```python
from build123d import *

# Parameters (mm, degrees)
BOSS_EXTRUDE1_DEPTH = 5
FILLET1_R           = 1


with BuildPart() as part:
    # Sketch1 → Boss-Extrude1 (new body)
    with BuildSketch(Plane.XY):
        Polygon((0, 0), (133, 0), (133, 12.3), (123.25, 12.3), (123.25, 10.3), (128.25, 10.3), (128.25, 5), (10, 5), (10, 10.3), (19, 10.3), (19, 30), (0, 30), align=None)
    extrude(amount=BOSS_EXTRUDE1_DEPTH)

    # Mirror1: part across plane


with BuildPart() as part_1:
    add(part.part)
    add(part.part.mirror(Plane(origin=(133, 12.3, 5), x_dir=(0, 0, 1), z_dir=(-1, 0, 0))))

    # Fillet1
    fillet1_edges = [part_1.edges().sort_by_distance(p)[0] for p in [
        (0, 30, 2.5),
        (19, 30, 2.5),
        (19, 10.3, 2.5),
        (0, 0, 2.5),
        (266, 0, 2.5),
        (247, 10.3, 2.5),
        (247, 30, 2.5),
        (266, 30, 2.5),
    ]]
    fillet(fillet1_edges, radius=FILLET1_R)


solid = part_1.part
```
Design review of the part built by this model. Coordinates are the model's own, in mm. A direction names the side the tool comes from. Give positions to 0.01 mm unless a question says otherwise; leave off trailing zeros. Loops run counter-clockwise (first coordinate to the right, second up) from the corner with the lowest first, then second, coordinate; pieces in that order, holes last. Notation, with made-up numbers: (48.25, -23) -> (58.25, -23) arc R22 ccw to (58.25, -11) -> close; hole circle Ø1 at (35.5, -3). An arc over 180 degrees is marked (long way). Write each question's results on one line, items separated by ' | '.
Q1. Machinability: for faces 1 (the face through (247, 20, 2)), 2 (the face through (134, 11, 5)), 3 (the face through (252, 10.3, 2)), which of the approach directions +Z, -Z, +X, -X, +Y, -Y give a long, thin tool a straight path to every point of the face, cutting with its end or side? Answer none if there is none.
Reply:
face 1: +Z, -Z, +Y | face 2: +Z, +X, -X, +Y, -Y | face 3: +Z, -Z
Q2. Take a section at B-B, the plane z = 1.15. Write out the cut boundary in (x, y).
Reply:
outline: (0, 1) arc R1 ccw to (1, 0) -> (265, 0) arc R1 ccw to (266, 1) -> (266, 29) arc R1 ccw to (265, 30) -> (248, 30) arc R1 ccw to (247, 29) -> (247, 11.3) arc R1 ccw to (248, 10.3) -> (256, 10.3) -> (256, 5) -> (137.75, 5) -> (137.75, 10.3) -> (142.75, 10.3) -> (142.75, 12.3) -> (123.25, 12.3) -> (123.25, 10.3) -> (128.25, 10.3) -> (128.25, 5) -> (10, 5) -> (10, 10.3) -> (18, 10.3) arc R1 ccw to (19, 11.3) -> (19, 29) arc R1 ccw to (18, 30) -> (1, 30) arc R1 ccw to (0, 29) -> close
Q3. Take a section at A-A, the plane y = 17. Write out the cut boundary in (x, z), plus the area to 3 significant figures.
Reply:
outline: (0, 0) -> (19, 0) -> (19, 5) -> (0, 5) -> close; (247, 0) -> (266, 0) -> (266, 5) -> (247, 5) -> close | area: 190 mm²
Q4. Wall thickness on L1, parallel to X at y = 8.5, z = 4; L2, parallel to X at y = 13.5, z = 2.05; L3, parallel to Y at x = 185, z = 1.2: over which ranges is each line inside the solid? List them lowest first.
Reply:
L1: x = 0 to 10, 128.25 to 137.75, 256 to 266 | L2: x = 0 to 19, 247 to 266 | L3: y = 0 to 5
Q5. The part is to be moulded in two halves that separate along Y. For faces 4 (the face through (140, 10.3, 2)), 5 (the face through (19, 20, 2)), 6 (the face through (256, 8, 2)), 7 (the face through (133, 12.3, 2)), say which applies: +Y half, -Y half, draft (parallel to the pull), parting line (faces both ways), or undercut.
Reply:
face 4: undercut | face 5: draft | face 6: undercut | face 7: +Y half
Q6. For pin 1 Ø1.5 at (x, z) = (175, 1.5) entering from +Y, flat-tipped, find the tip position at first contact; note if it passes through.
Reply:
pin 1: stops at y = 5
Q7. Take a section at C-C, the plane x = 161. Write out the cut boundary in (y, z).
Reply:
outline: (0, 0) -> (5, 0) -> (5, 5) -> (0, 5) -> close
